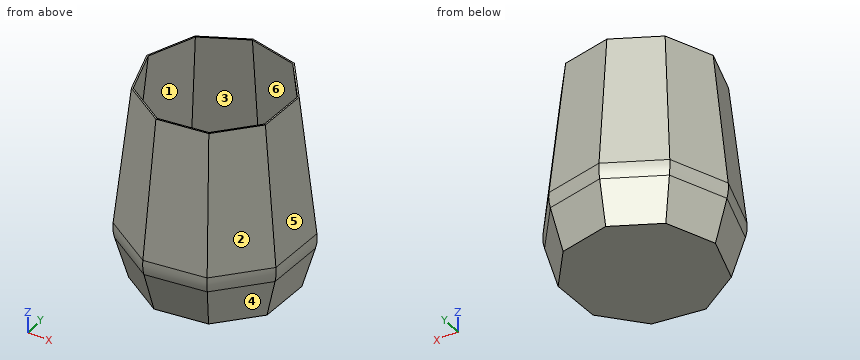
from build123d import *

# Parameters (mm, degrees)
SALIENTE_EXTRUIR4_DEPTH = 35
SALIENTE_EXTRUIR4_DRAFT = -15
SALIENTE_EXTRUIR5_DEPTH = 104
SALIENTE_EXTRUIR5_DRAFT = -6
REDONDEO1_R             = 30
VACIADO1_T              = -1


with BuildPart() as part:
    # Croquis1 → Saliente-Extruir4 (with draft: the straight prism first)
    with BuildSketch(Plane.XY):
        Polygon((23.773844097, -47.265828947), (48.59371037, -20.926193194), (50.676039503, 15.205040923), (29.04648655, 44.221667407), (-6.174240275, 52.546484242), (-38.505971456, 36.284217111), (-52.820330647, 3.04416154), (-42.419470096, -31.620291048), (-12.170068047, -51.489258034), align=None)
    extrude(amount=SALIENTE_EXTRUIR4_DEPTH)
    # Saliente-Extruir4: the draft: its side faces are tilted about the plane it starts from
    saliente_extruir4_sides = [part.faces().sort_by_distance(p)[0] for p in [
        (36.183777233, -34.09601107, 17.5),
        (49.634874936, -2.860576136, 17.5),
        (39.861263027, 29.713354165, 17.5),
        (11.436123138, 48.384075824, 17.5),
        (-22.340105865, 44.415350676, 17.5),
        (-45.663151051, 19.664189326, 17.5),
        (-47.619900371, -14.288064754, 17.5),
        (-27.294769071, -41.554774541, 17.5),
        (5.801888025, -49.37754349, 17.5),
    ]]
    draft(saliente_extruir4_sides, Plane.XY, SALIENTE_EXTRUIR4_DRAFT)


with BuildPart() as saliente_extruir5_tool:
    # Croquis12 → Saliente-Extruir5 (with draft: the straight prism first)
    with BuildSketch(Plane(origin=(0, 0, 35), x_dir=(-1, 0, 0), z_dir=(0, 0, -1))):
        Polygon((50.42110527, -37.584864214), (62.783892537, 3.618385358), (45.76939872, 43.128552207), (7.338894572, 62.458390158), (-34.525559909, 52.563253206), (-60.235121199, 18.073185904), (-57.759999842, -24.873525944), (-28.258332628, -56.181638564), (14.465722479, -61.201738111), align=None)
    extrude(amount=-SALIENTE_EXTRUIR5_DEPTH)
    # Saliente-Extruir5: the draft: its side faces are tilted about the plane it starts from
    saliente_extruir5_sides = [saliente_extruir5_tool.faces().sort_by_distance(p)[0] for p in [
        (-56.602498903, -16.983239428, 87),
        (-54.276645628, 23.373468782, 87),
        (-26.554146646, 52.793471182, 87),
        (13.593332668, 57.510821682, 87),
        (47.380340554, 35.318219555, 87),
        (58.997560521, -3.40017002, 87),
        (43.009166235, -40.527582254, 87),
        (6.896305074, -58.691688337, 87),
        (-32.443413875, -49.393301163, 87),
    ]]
    draft(saliente_extruir5_sides, Plane(origin=(0, 0, 35), x_dir=(-1, 0, 0), z_dir=(0, 0, -1)), SALIENTE_EXTRUIR5_DRAFT)


with BuildPart() as part_1:
    add(part.part)

    # Saliente-Extruir5: add saliente_extruir5_tool
    add(saliente_extruir5_tool.part)

    # Redondeo1
    redondeo1_edges = [part_1.edges().sort_by_distance(p)[0] for p in [
        (13.593332668, 57.510821682, 35),
        (-26.554146646, 52.793471182, 35),
        (-54.276645628, 23.373468782, 35),
        (-56.602498903, -16.983239428, 35),
        (-32.443413875, -49.393301163, 35),
        (6.896305074, -58.691688337, 35),
        (43.009166235, -40.527582254, 35),
        (58.997560521, -3.40017002, 35),
        (47.380340554, 35.318219555, 35),
    ]]
    fillet(redondeo1_edges, radius=REDONDEO1_R)

    # Vaciado1
    vaciado1_openings = [part_1.faces().sort_by_distance(p)[0] for p in [
        (0, 0, 139),
    ]]
    offset(amount=VACIADO1_T, openings=vaciado1_openings)


solid = part_1.part
CAD build for the part. Positions are in the model's coordinates, mm. Face numbers are marked on the shaded views. A direction names the side the tool comes from. Give positions to 0.01 mm unless a question says otherwise; leave off trailing zeros. Loops run counter-clockwise (first coordinate to the right, second up) from the corner with the lowest first, then second, coordinate; pieces in that order, holes last. Notation, with made-up numbers: M -37.75,84.25 L -25.75,84.25 A20 cw -25.75,115.25 Z; hole C 89.25,-8 d11. An arc over 180 degrees is marked long. Answer in a Markdown table with one row per item. Add a question column.
Item 1: Band-saw the part on B-B on z = 66. Give the cut face in (x, y), then the cut area to 3 significant figures.
Item 2: Tool access for the marked faces 1 and 2: list every direction of +Z, -Z, +X, -X, +Y, -Y with a clear straight run to the whole face (end or side of a thin tool).
Item 3: Probe probe 1 along Z at (x, y) = (11, -24.5); probe 2 along Y at (x, z) = (19.5, 46); probe 3 along X at (y, z) = (12, 61). List the from-to ranges inside material, lowest first.
Item 4: Band-saw the part on A-A on z = 82. Give the cut face in (x, y), then the cut area to 3 significant figures.
Item 5: Drop flat-ended pins along their axis: P1, Ø10, axis at x = 15, z = 66, coming from the -Y side; P2, Ø10, axis at x = 31.5, z = 62.5, coming from the -Y side; P3, Ø4, axis at x = -20, y = 32.5, coming from the +Z side. Give the stop position or say it passes through.
Item 6: Mould opens along Z. For the marked faces 3, 4, 5 and 6 say: +Z half, -Z half, draft (parallel to the pull), parting line (faces both ways), or undercut.
Reply:
| question | item | result |
|---|---|---|
| 1 | outline | M -59.32,3.42 L -47.64,-35.51 L -13.67,-57.83 L 26.7,-53.08 L 54.58,-23.5 L 56.91,17.08 L 32.62,49.67 L -6.93,59.01 L -43.25,40.75 Z; hole M -58.25,3.36 L -46.78,-34.87 L -13.42,-56.79 L 26.22,-52.13 L 53.59,-23.08 L 55.89,16.77 L 32.03,48.77 L -6.81,57.95 L -42.47,40.02 Z |
| 1 | area | 365 mm^2 |
| 2 | face 1 | none |
| 2 | face 2 | +Z, +X, -Y |
| 3 | probe 1 | z = 0 to 1 |
| 3 | probe 2 | y = -56.05 to -55.03, 53.89 to 54.93 |
| 3 | probe 3 | x = -56.2 to -55.1, 56.14 to 57.15 |
| 4 | outline | M -57.54,3.32 L -46.21,-34.44 L -13.26,-56.09 L 25.9,-51.49 L 52.93,-22.79 L 55.2,16.56 L 31.64,48.17 L -6.73,57.24 L -41.94,39.52 Z; hole M -56.47,3.25 L -45.35,-33.8 L -13.01,-55.04 L 25.42,-50.53 L 51.95,-22.37 L 54.18,16.25 L 31.05,47.28 L -6.6,56.17 L -41.16,38.79 Z |
| 4 | area | 353 mm^2 |
| 5 | P1 | stops at y = -55.25 |
| 5 | P2 | stops at y = -53.65 |
| 5 | P3 | stops at z = 1 |
| 6 | face 3 | undercut |
| 6 | face 4 | -Z half |
| 6 | face 5 | +Z half |
| 6 | face 6 | undercut |
